Autodesk Inventor part; units mm, degrees
ref_plane "YZ Plane" through (0, 0, 0) normal (1, 0, 0) x (0, 1, 0)
ref_plane "XZ Plane" through (0, 0, 0) normal (0, 1, 0) x (-1, 0, 0)
ref_plane "XY Plane" through (0, 0, 0) normal (0, 0, 1) x (1, 0, 0)
sketch "Profile" plane through (0, 0, 0) normal (0, 0, 1) x (1, 0, 0)
  line L0 (0, 0) -> (0, 330.2)
  line L1 (0, 0) -> (152.4, 0)
  line L2 (152.4, 0) -> (152.4, 342.9)
  line L3 (152.4, 342.9) -> (139.7, 342.9) construction
  line L4 (152.4, 342.9) -> (139.7, 342.9) construction
  arc A0 (152.4, 342.9) -> (137.4098, 355.3918) centre (139.7, 342.9) ccw
  line L5 (0, 330.2) -> (137.4098, 355.3918)
  dimension "d0" = 330.2
  dimension "d1" = 152.4
  dimension "d2" = 342.9
  dimension "d3" = 12.7
  dimension "d4" = 12.7
sketch "Sketch1" plane through (0, 0, 0) normal (1, 0, 0) x (0, 1, 0)
  line L0 (0, 0) -> (0, 330.2)
  line L1 (0, 0) -> (152.4, 0)
  line L2 (152.4, 0) -> (152.4, 342.9)
  line L3 (152.4, 342.9) -> (139.7, 342.9) construction
  line L4 (152.4, 342.9) -> (139.7, 342.9) construction
  arc A0 (152.4, 342.9) -> (137.4098, 355.3918) centre (139.7, 342.9) ccw
  line L5 (0, 330.2) -> (137.4098, 355.3918)
extrude "Extrusion1" add sketch "Sketch1" along normal blind 1647.825
properties part number "D" material "Granite, Cut, Polished"
The model under review builds one solid part; all positions refer to its coordinate system, in mm. Coordinates: 2 decimals unless noted, no trailing zeros. Loops run counter-clockwise (first coordinate to the right, second up) from the corner with the lowest first, then second, coordinate; pieces in that order, holes last. Notation, with made-up numbers: M -32.5,-37.5 L -2.5,-37.5 A20 ccw -2.5,-33.5 Z; hole C 54.5,67.25 d10. An arc over 180 degrees is marked long. Put each result on its own line as item: value. Start each with the question number.
Q1. Wall thickness on line 1 (Z direction, x = 333.5, y = 119); line 2 (Z direction, x = 1254.5, y = 125.5): over which ranges is each line inside the solid? List them lowest first.
Q2. Add section C-C (y = 100). Write out the cut boundary in (x, z) (3 decimals), and give its area (3 significant figures).
Q3. Add section A-A (y = 39). Write out the cut boundary in (x, z) (3 decimals).
Q4. Clearance check with flat-ended pins moving along their axes: pin 1 (4 mm diameter, centred on x = 274, y = 121, fed in from +Z); pin 2 (1.5 mm diameter, centred on x = 272.5, y = 63, fed in from -Z). State where each tip first meets the part, or that it passes through.
Q5. Add section B-B (x = 991.5). Write out the cut boundary in (y, z).
Answers:
1. line 1: z = 0 to 352.02
1. line 2: z = 0 to 353.21
2. outline: M 0,0 L 1647.825,0 L 1647.825,348.533 L 0,348.533 Z
2. area: 574,000 mm^2
3. outline: M 0,0 L 1647.825,0 L 1647.825,337.35 L 0,337.35 Z
4. pin 1: stops at z = 352.75
4. pin 2: stops at z = 0
5. outline: M 0,0 L 152.4,0 L 152.4,342.9 A12.7 ccw 137.41,355.39 L 0,330.2 Z
